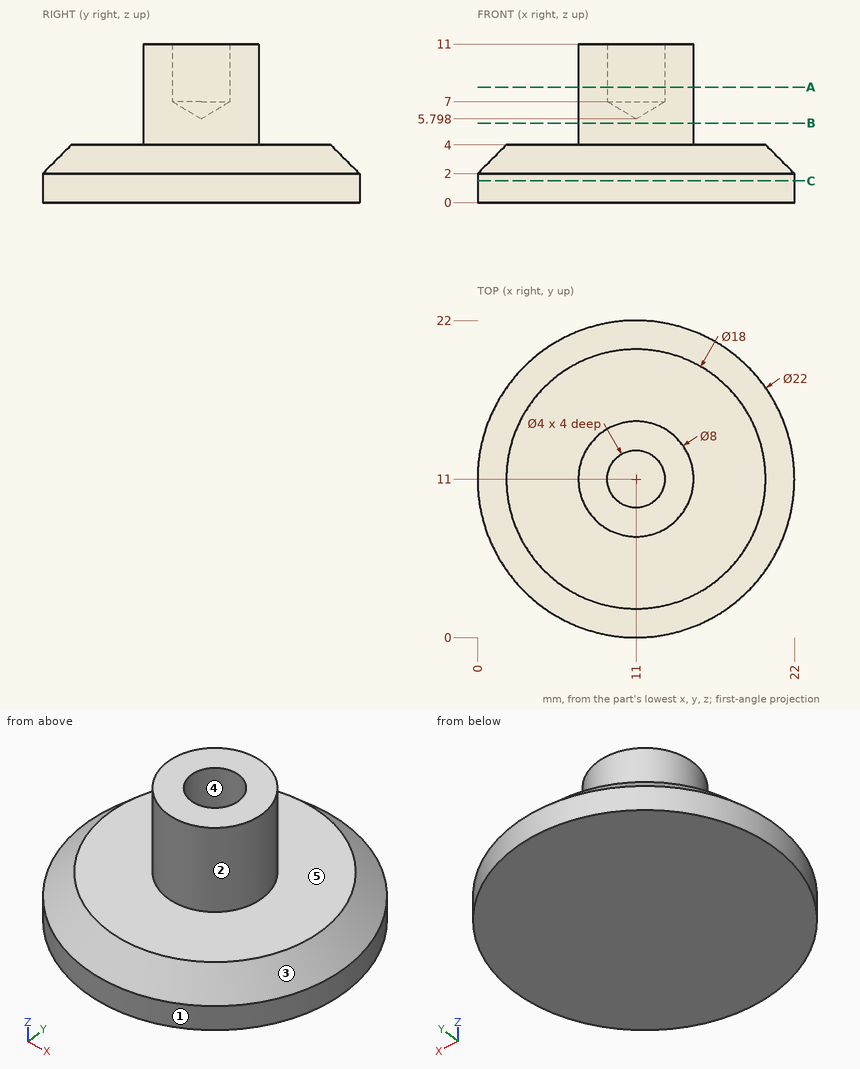
Here's the drawing with two shaded views (mm, measured from the low corner). I have some questions. A direction names the side the tool comes from. Coordinates: 2 decimals unless noted, no trailing zeros. Order: outer loops, then holes, each group sorted by start corner. A loop starts at its lowest first (then second) coordinate and runs counter-clockwise, first axis right, second up. Notation, with made-up numbers: (61.25, 32.5) - (102.25, 32.5) arc R22 cw to (102.25, 65.5) - close; hole circle Ø7 at (60.25, -18). An arc over 180 degrees is marked (long way). Answer in a Markdown table with one row per item. Add a question column.
(1) I need wall thicknesses on L1, parallel to Y at x = 11, z = 9.3; L2, parallel to Z at x = 6.5, y = 16.25; L3, parallel to Z at x = 4.5, y = 17.5. Which ranges of each line are inside material? Lowest first, please.
(2) If we mould it in two halves opening along Y, with no side actions, what happens to the marked faces 3, 4 and 5? For each: released by +Y, released by -Y, zero draft, split by the parting line, or undercut.
(3) If we section it at B-B, the plane z = 5.5: Please give me the cut outline in (x, y), then the cut area to 3 significant figures.
(4) If we section it at C-C, the plane z = 1.5: Please give me the cut outline in (x, y).
(5) If we section it at A-A, the plane z = 8: Please give me the cut outline in (x, y).
(6) Will these pins go through, and if not, where does the flat tip stop? pin 1 (5 mm diameter, centred on x = 12, z = 5.5, fed in from -Y); pin 2 (4 mm diameter, centred on x = 9.5, z = 9, fed in from -Y); pin 3 (1.5 mm diameter, centred on x = 19, y = 12, fed in from +Z).
(7) On a 3-axis mill with a long thin cutter (end or side, diameter ignored), from which of +Z, -Z, +X, -X, +Y, -Y can I reach the whole of each face in a straight line? I mean the marked faces 1 and 2. Say none if no direction works.
Results are:
| question | item | result |
|---|---|---|
| 1 | L1 | y = 7 to 9, 13 to 15 |
| 1 | L2 | z = 0 to 4 |
| 1 | L3 | z = 0 to 3.81 |
| 2 | face 3 | split by the parting line |
| 2 | face 4 | undercut |
| 2 | face 5 | zero draft |
| 3 | outline | circle Ø8 at (11, 11) |
| 3 | area | 50.3 mm2 |
| 4 | outline | circle Ø22 at (11, 11) |
| 5 | outline | circle Ø8 at (11, 11); hole circle Ø4 at (11, 11) |
| 6 | pin 1 | stops at y = 1.04 |
| 6 | pin 2 | stops at y = 7 |
| 6 | pin 3 | stops at z = 4 |
| 7 | face 1 | +Z, -Z |
| 7 | face 2 | +Z |
